Verification items for the finished model (mm, model axes). Give positions to 0.01 mm unless a question says otherwise; leave off trailing zeros. Loops run counter-clockwise (first coordinate to the right, second up) from the corner with the lowest first, then second, coordinate; pieces in that order, holes last. Notation, with made-up numbers: (-10.75, 19) - (-4.75, 19) arc R21 ccw to (-4.75, 48) - close; hole circle Ø3 at (4.25, -13). An arc over 180 degrees is marked (long way). One line per item, written item: value. Start each with the question number.
1. Sectioned sample at A-A (x = 0). Record the cut outline in (y, z).
2. Scan lines: L1, parallel to X at y = 0.6, z = -15.5; L2, parallel to Z at x = -26, y = 1; L3, parallel to Z at x = 13, y = 0.65. Record each from-to range of solid material in increasing order. Write a range as [from, to].
3. Gauge pin test, flat ends, axial feed: pin 1 (2.5 mm diameter, centred on x = -25.5, z = -44.17, fed in from +Y); pin 2 (1 mm diameter, centred on x = 108.5, y = 1.5, fed in from +Z). Record the tip position at first contact, or that the pin passes through.
4. Sectioned sample at B-B (z = 51). Record the cut outline in (x, y), plus the area to 3 significant figures.
5. Sectioned sample at D-D (z = -6.5). Record the cut outline in (x, y).
6. Sectioned sample at C-C (y = 1.3). Count the separate pieces of the cut face and the enclosed holes in it, plus the area to 3 significant figures.
from build123d import *

# Parameters (mm, degrees)
SKETCH1_R           = 57.5
BOSS_EXTRUDE1_DEPTH = 3
SKETCH2_W           = 140
SKETCH2_H           = 70
BOSS_EXTRUDE2_DEPTH = 3
BOSS_EXTRUDE3_DEPTH = 3
SKETCH4_R           = 43
CUT_EXTRUDE1_DEPTH  = 4
SKETCH7_R           = 3.25
CUT_EXTRUDE8_DEPTH  = 4
LPATTERN1_COUNT     = 3
LPATTERN1_PITCH     = 20
CUT_EXTRUDE5_START  = -1
SKETCH5_R           = 2.25
CUT_EXTRUDE5_DEPTH  = 5
CIRPATTERN1_COUNT   = 12
SKETCH12_R          = 4.5
CUT_EXTRUDE17_DEPTH = 4
CIRPATTERN2_COUNT   = 4
SKETCH13_R          = 3.25
CUT_EXTRUDE18_DEPTH = 10
LPATTERN2_COUNT     = 3
LPATTERN2_PITCH     = 20


with BuildPart() as part:
    # Sketch1 → Boss-Extrude1 (new body)
    with BuildSketch(Plane(origin=(0, 0, 0), x_dir=(1, 0, 0), z_dir=(0, 1, 0))):
        Circle(SKETCH1_R)
    extrude(amount=BOSS_EXTRUDE1_DEPTH)

    # Sketch2 → Boss-Extrude2 (add)
    with BuildSketch(Plane(origin=(0, 0, 0), x_dir=(1, 0, 0), z_dir=(0, 1, 0))):
        with Locations((63.125798099, 0)):
            Rectangle(SKETCH2_W, SKETCH2_H)
    extrude(amount=BOSS_EXTRUDE2_DEPTH)

    # Sketch3 → Boss-Extrude3 (add)
    with BuildSketch(Plane(origin=(0, 0, 0), x_dir=(1, 0, 0), z_dir=(0, 1, 0))):
        Polygon((89.373258538, 35), (13.76852627, 55.827212758), (13.76852627, 13.558751548), align=None)
    extrude(amount=BOSS_EXTRUDE3_DEPTH)

    # Sketch4 → Cut-Extrude1 (cut, through all)
    with BuildSketch(Plane(origin=(0, 3, 0), x_dir=(1, 0, 0), z_dir=(0, 1, 0))):
        Circle(SKETCH4_R)
    extrude(amount=-CUT_EXTRUDE1_DEPTH, mode=Mode.SUBTRACT)

    # Sketch7 → Cut-Extrude8 (cut, through all)
    with BuildSketch(Plane(origin=(0, 3, 0), x_dir=(1, 0, 0), z_dir=(0, 1, 0))):
        with Locations((123.125798099, 15)):
            Circle(SKETCH7_R)
        with Locations((123.125798099, -15)):
            Circle(SKETCH7_R)
    cut_extrude8 = extrude(amount=-CUT_EXTRUDE8_DEPTH, mode=Mode.SUBTRACT)

    # LPattern1: Cut-Extrude8 ×3
    with Locations(*[(-i * LPATTERN1_PITCH, 0, 0) for i in range(1, LPATTERN1_COUNT)]):
        add(cut_extrude8, mode=Mode.SUBTRACT)

    # Sketch5 → Cut-Extrude5 (cut)
    with BuildSketch(Plane(origin=(0, 0, 0), x_dir=(1, 0, 0), z_dir=(0, 1, 0)).offset(CUT_EXTRUDE5_START)):
        with Locations((-51, 0)):
            Circle(SKETCH5_R)
    cut_extrude5 = extrude(amount=CUT_EXTRUDE5_DEPTH, mode=Mode.SUBTRACT)

    # CirPattern1: Cut-Extrude5 ×12 about axis
    cirpattern1_axis = Axis((0, 0, 0), (0, 1, 0))
    for i in range(1, CIRPATTERN1_COUNT):
        add(cut_extrude5.rotate(cirpattern1_axis, i * 360 / CIRPATTERN1_COUNT), mode=Mode.SUBTRACT)

    # Sketch12 → Cut-Extrude17 (cut, through all)
    with BuildSketch(Plane(origin=(0, 3, 0), x_dir=(1, 0, 0), z_dir=(0, 1, 0))):
        with Locations((-49.262217141, 13.1997713)):
            Circle(SKETCH12_R)
    cut_extrude17 = extrude(amount=-CUT_EXTRUDE17_DEPTH, mode=Mode.SUBTRACT)

    # CirPattern2: Cut-Extrude17 ×4 about axis
    cirpattern2_axis = Axis((0, 0, 0), (0, 1, 0))
    for i in range(1, CIRPATTERN2_COUNT):
        add(cut_extrude17.rotate(cirpattern2_axis, i * 360 / CIRPATTERN2_COUNT), mode=Mode.SUBTRACT)

    # Sketch13 → Cut-Extrude18 (cut)
    with BuildSketch(Plane(origin=(0, 3, 0), x_dir=(1, 0, 0), z_dir=(0, 1, 0))):
        with Locations((123.125798099, 0)):
            Circle(SKETCH13_R)
    cut_extrude18 = extrude(amount=-CUT_EXTRUDE18_DEPTH, mode=Mode.SUBTRACT)

    # LPattern2: Cut-Extrude18 ×3
    with Locations(*[(-i * LPATTERN2_PITCH, 0, 0) for i in range(1, LPATTERN2_COUNT)]):
        add(cut_extrude18, mode=Mode.SUBTRACT)


solid = part.part
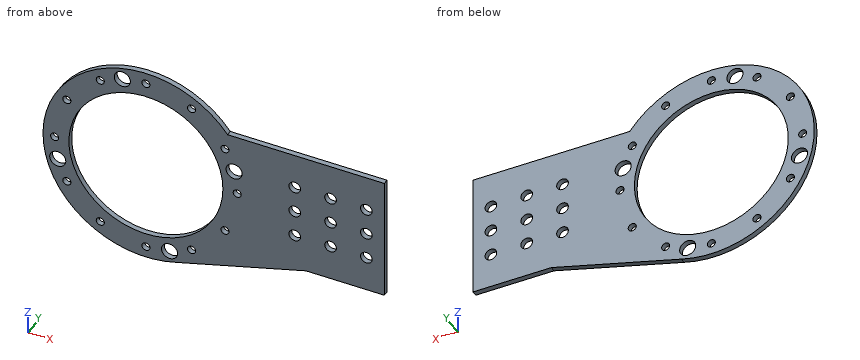
Results are:
1. outline: (0, -57.5) - (3, -57.5) - (3, -53.25) - (0, -53.25) - close; (0, -48.75) - (3, -48.75) - (3, -43) - (0, -43) - close; (0, 43) - (3, 43) - (3, 48.75) - (0, 48.75) - close; (0, 53.25) - (3, 53.25) - (3, 57.5) - (0, 57.5) - close
2. L1: x = [-55.37, -53.13], [-45.39, -40.11], [40.11, 79.91], [86.34, 99.91], [106.34, 119.91], [126.34, 133.13]
2. L2: z = [-51.29, -46.36], [-41.97, -34.25], [34.25, 41.97], [46.36, 51.29]
2. L3: z = [-56.01, -53.76], [-44.77, -40.99], [40.99, 56.01]
3. pin 1: passes through
3. pin 2: stops at z = 35
4. outline: (-26.56, 0) - (-17.35, 0) - (-17.35, 3) - (-26.56, 3) - close; (-9.05, 0) - (-2.25, 0) - (-2.25, 3) - (-9.05, 3) - close; (2.25, 0) - (26.56, 0) - (26.56, 3) - (2.25, 3) - close
4. area: 121 mm^2
5. outline: (-57.13, 0) - (-42.51, 0) - (-42.51, 3) - (-57.13, 3) - close; (42.51, 0) - (133.13, 0) - (133.13, 3) - (42.51, 3) - close
6. separate pieces: 1
6. enclosed holes: 26
6. area: 9,770 mm^2
